Part model, mm, in its own coordinate system. A direction names the side the tool comes from. Round coordinates to 2 decimals unless told otherwise and drop trailing zeros. Write each loop counter-clockwise with the first axis right and the second up, starting at its lowest first coordinate (ties: lowest second). Pieces come first, ordered by that corner, then holes. Notation, with made-up numbers: M -36,-23 L 21,-23 A15 ccw 21,-2 Z; hole C 8,45.25 d7. An arc over 180 degrees is marked long. One line per question, with ' | ' between items. Start each with the question number.
1) Tool access for faces 1 (the face through (-28, 16.816, 2)), 2 (the face through (-34, 46.816, 2)): list every direction of +Z, -Z, +X, -X, +Y, -Y with a clear straight run to the whole face (end or side of a thin tool).
2) Wall check: probe 1 along Y at (x, z) = (-56.5, 2.5); probe 2 along Y at (x, z) = (-64.5, 4.5); probe 3 along X at (y, z) = (17.5, 4.45). Give the ranges that are in metal, low to high. Write a range as [from, to].
3) Saw through at A-A (x = -21.5). List the corners of the cut face in (y, z).
4) Mould opens along X. For faces 3 (the face through (-2.86, 30.66, 2.46)), 4 (the face through (-7, 16.816, 2)), 5 (the face through (12.204, 27, 2)), 6 (the face through (-34.5, 27.1, 0)) say: pulls with the +X half, pulls with the -X half, needs draft (parallel to the pull), parting line crosses it, or undercut.
5) Saw through at B-B (z = 1.7). Give the number of separate pieces and of enclosed holes in the cut face, plus the area to 3 significant figures.
```python
from build123d import *

# Parameters (mm, degrees)
F0_W     = 92.1527777778
F0_H     = 40
F1_DEPTH = 5
F2_R     = 4


with BuildPart() as f1:
    # F0 (on Top) → F1 (new body)
    with BuildSketch(Plane.XY):
        with Locations((-33.8721656561, 26.8162500644)):
            Rectangle(F0_W, F0_H)
        with BuildLine():
            add(Edge.make_bspline(
                [(-54.2280684339, 33.8127778422), (-56.4806726005, 34.8674653422), (-58.7332767672, 34.8674653422)],
                knots=[0, 0, 0, 1, 1, 1], degree=2))
            add(Edge.make_bspline(
                [(-58.7332767672, 34.8674653422), (-62.0015059339, 34.8674653422), (-63.893867045, 32.6908160367)],
                knots=[0, 0, 0, 1, 1, 1], degree=2))
            add(Edge.make_bspline(
                [(-63.893867045, 32.6908160367), (-65.7862281561, 30.5141667311), (-65.7862281561, 26.7294445089)],
                knots=[0, 0, 0, 1, 1, 1], degree=2))
            add(Edge.make_bspline(
                [(-65.7862281561, 26.7294445089), (-65.7862281561, 22.84055562), (-63.9611413505, 20.7159896478)],
                knots=[0, 0, 0, 1, 1, 1], degree=2))
            add(Edge.make_bspline(
                [(-63.9611413505, 20.7159896478), (-62.136054545, 18.5914236756), (-58.7593184339, 18.5914236756)],
                knots=[0, 0, 0, 1, 1, 1], degree=2))
            add(Edge.make_bspline(
                [(-58.7593184339, 18.5914236756), (-56.6846656561, 18.5914236756), (-54.0240753783, 19.3379514533)],
                knots=[0, 0, 0, 1, 1, 1], degree=2))
            Line((-54.0240753783, 19.3379514533), (-54.0240753783, 17.3197222867))
            add(Edge.make_bspline(
                [(-54.0240753783, 17.3197222867), (-56.0857073228, 16.5428125644), (-59.1108809339, 16.5428125644)],
                knots=[0, 0, 0, 1, 1, 1], degree=2))
            add(Edge.make_bspline(
                [(-59.1108809339, 16.5428125644), (-63.4902212117, 16.5428125644), (-65.8708635728, 19.2034028422)],
                knots=[0, 0, 0, 1, 1, 1], degree=2))
            add(Edge.make_bspline(
                [(-65.8708635728, 19.2034028422), (-68.2515059339, 21.86399312), (-68.2515059339, 26.7598264533)],
                knots=[0, 0, 0, 1, 1, 1], degree=2))
            add(Edge.make_bspline(
                [(-68.2515059339, 26.7598264533), (-68.2515059339, 29.8240625644), (-67.1056726005, 32.1287500644)],
                knots=[0, 0, 0, 1, 1, 1], degree=2))
            add(Edge.make_bspline(
                [(-67.1056726005, 32.1287500644), (-65.9598392672, 34.4334375644), (-63.796210795, 35.6812674256)],
                knots=[0, 0, 0, 1, 1, 1], degree=2))
            add(Edge.make_bspline(
                [(-63.796210795, 35.6812674256), (-61.6325823228, 36.9290972867), (-58.7028948228, 36.9290972867)],
                knots=[0, 0, 0, 1, 1, 1], degree=2))
            add(Edge.make_bspline(
                [(-58.7028948228, 36.9290972867), (-55.5865753783, 36.9290972867), (-53.2515059339, 35.7919445089)],
                knots=[0, 0, 0, 1, 1, 1], degree=2))
            Line((-53.2515059339, 35.7919445089), (-54.2280684339, 33.8127778422))
        make_face(mode=Mode.SUBTRACT)
        with BuildLine():
            Line((-37.0275476005, 36.6469792311), (-34.7228601005, 36.6469792311))
            Line((-34.7228601005, 36.6469792311), (-34.7228601005, 23.81711812))
            add(Edge.make_bspline(
                [(-34.7228601005, 23.81711812), (-34.7228601005, 20.4230208978), (-36.7714712117, 18.4829167311)],
                knots=[0, 0, 0, 1, 1, 1], degree=2))
            add(Edge.make_bspline(
                [(-36.7714712117, 18.4829167311), (-38.8200823228, 16.5428125644), (-42.4008114894, 16.5428125644)],
                knots=[0, 0, 0, 1, 1, 1], degree=2))
            add(Edge.make_bspline(
                [(-42.4008114894, 16.5428125644), (-45.9815406561, 16.5428125644), (-47.9411760728, 18.4981077033)],
                knots=[0, 0, 0, 1, 1, 1], degree=2))
            add(Edge.make_bspline(
                [(-47.9411760728, 18.4981077033), (-49.9008114894, 20.4534028422), (-49.9008114894, 23.8692014533)],
                knots=[0, 0, 0, 1, 1, 1], degree=2))
            Line((-49.9008114894, 23.8692014533), (-49.9008114894, 36.6469792311))
            Line((-49.9008114894, 36.6469792311), (-47.5917837117, 36.6469792311))
            Line((-47.5917837117, 36.6469792311), (-47.5917837117, 23.7086111756))
            add(Edge.make_bspline(
                [(-47.5917837117, 23.7086111756), (-47.5917837117, 21.2259722867), (-46.2354469061, 19.8956771478)],
                knots=[0, 0, 0, 1, 1, 1], degree=2))
            add(Edge.make_bspline(
                [(-46.2354469061, 19.8956771478), (-44.8791101005, 18.5653820089), (-42.2489017672, 18.5653820089)],
                knots=[0, 0, 0, 1, 1, 1], degree=2))
            add(Edge.make_bspline(
                [(-42.2489017672, 18.5653820089), (-39.7402212117, 18.5653820089), (-38.3838844061, 19.9021875644)],
                knots=[0, 0, 0, 1, 1, 1], degree=2))
            add(Edge.make_bspline(
                [(-38.3838844061, 19.9021875644), (-37.0275476005, 21.23899312), (-37.0275476005, 23.7346528422)],
                knots=[0, 0, 0, 1, 1, 1], degree=2))
            Line((-37.0275476005, 23.7346528422), (-37.0275476005, 36.6469792311))
        make_face(mode=Mode.SUBTRACT)
        Polygon((-23.425117045, 28.0315278422), (-15.1525476005, 16.8162500644), (-17.8652212117, 16.8162500644), (-25.0917837117, 26.43430562), (-27.1707767672, 24.5896875644), (-27.1707767672, 16.8162500644), (-29.4754642672, 16.8162500644), (-29.4754642672, 36.6469792311), (-27.1707767672, 36.6469792311), (-27.1707767672, 26.8119097867), (-18.1777212117, 36.6469792311), (-15.4520267672, 36.6469792311), align=None, mode=Mode.SUBTRACT)
        Polygon((-12.6308462117, 36.6469792311), (-7.3791101005, 26.7294445089), (-2.0926517672, 36.6469792311), (0.403007955, 36.6469792311), (-6.2159156561, 24.5072222867), (-6.2159156561, 16.8162500644), (-8.5466448228, 16.8162500644), (-8.5466448228, 24.3987153422), (-15.1525476005, 36.6469792311), align=None, mode=Mode.SUBTRACT)
    extrude(amount=F1_DEPTH)

    # F2
    f2_edges = [f1.edges().sort_by_distance(p)[0] for p in [
        (-79.948555, 46.81625, 2.5),
        (-79.948555, 6.81625, 2.5),
        (12.204223, 6.81625, 2.5),
        (12.204223, 46.81625, 2.5),
    ]]
    fillet(f2_edges, radius=F2_R)


solid = f1.part
```
Answer key:
1) face 1: +Z, -Z | face 2: +Z, -Z, +X, -X, +Y
2) probe 1: y = [6.82, 16.71], [18.78, 34.61], [36.77, 46.82] | probe 2: y = [6.82, 18], [21.44, 31.88], [35.23, 46.82] | probe 3: x = [-79.95, -63.65], [-54.02, -46.62], [-38.13, -29.48], [-27.17, -18.38], [-15.66, -8.55], [-6.22, 12.2]
3) outline: M 6.82,0 L 21.65,0 L 21.65,5 L 6.82,5 Z; M 25.42,0 L 30.11,0 L 30.11,5 L 25.42,5 Z; M 33.01,0 L 46.82,0 L 46.82,5 L 33.01,5 Z
4) face 3: undercut | face 4: undercut | face 5: pulls with the +X half | face 6: needs draft
5) separate pieces: 1 | enclosed holes: 4 | area: 3,300 mm2
